Solid Edge part; units mm, degrees
sketch "Sketch1" plane through (0, 0, 0) normal (0, 0, 1) x (1, 0, 0)
  circle A0 centre (0, 0) radius 32
  circle A1 centre (0, 0) radius 21.1
  circle A2 centre (27, 0) radius 1.7
  circle A3 centre (0, 27) radius 1.7
  circle A4 centre (-27, 0) radius 1.7
  circle A5 centre (0, -27) radius 1.7
extrude "Protrusion1" add sketch "Sketch1" along normal blind 7.15
sketch "Sketch2" plane through (0, 0, 7.15) normal (0, 0, 1) x (1, 0, 0)
  circle A0 centre (0, 0) radius 32
  circle A1 centre (0, 0) radius 17.5
  circle A2 centre (27, 0) radius 1.7
  circle A3 centre (0, 27) radius 1.7
  circle A4 centre (-27, 0) radius 1.7
  circle A5 centre (0, -27) radius 1.7
extrude "ExtrudedProtrusion_2" add sketch "Sketch2" along normal blind 14.7
sketch "Sketch3" plane through (0, 0, 21.85) normal (0, 0, 1) x (1, 0, 0)
  circle A0 centre (0, 0) radius 32
  circle A1 centre (0, 0) radius 21.1
  circle A2 centre (27, 0) radius 1.7
  circle A3 centre (0, 27) radius 1.7
  circle A4 centre (-27, 0) radius 1.7
  circle A5 centre (0, -27) radius 1.7
extrude "ExtrudedProtrusion_3" add sketch "Sketch3" along normal blind 7.15
sketch "Sketch4" plane through (0, 0, 18.5) normal (0, 0, 1) x (1, 0, 0)
  circle A0 centre (0, 0) radius 42
  circle A1 centre (0, 0) radius 17.5
  circle A2 centre (27, 0) radius 1.7
  circle A3 centre (0, 27) radius 1.7
  circle A4 centre (-27, 0) radius 1.7
  circle A5 centre (0, -27) radius 1.7
  circle A6 centre (37, 0) radius 1.7
  circle A7 centre (0, 37) radius 1.7
  circle A8 centre (-37, 0) radius 1.7
  circle A9 centre (0, -37) radius 1.7
extrude "ExtrudedProtrusion_4" add sketch "Sketch4" along normal blind 5
For this review, take the finished solid that the model builds, in its own axes (mm). A direction names the side the tool comes from. Round coordinates to 2 decimals unless told otherwise and drop trailing zeros. Order: outer loops, then holes, each group sorted by start corner. A loop starts at its lowest first (then second) coordinate and runs counter-clockwise, first axis right, second up. Notation, with made-up numbers: M 58,-13.5 L 101,-13.5 A20 ccw 101,8.5 Z; hole C 44,83.5 d5. An arc over 180 degrees is marked long. Write each question's results on one line, items separated by ' | '. Start each with the question number.
1. Add section D-D (y = 0). State how many separate pieces and enclosed holes the cut face has, then the cut area to 3 significant figures.
2. Draft analysis for pull direction Y (two halves, no side actions). For faces 1 (the face through (20.126, -6.338, 3.525)), 2 (the face through (-6.94, 31.24, 9.12)), 3 (the face through (-8, 16, 7.15)), 4 (the face through (9, -31, 23.5)), state which applies: pulls with the +Y half, pulls with the -Y half, needs draft (parallel to the pull), parting line crosses it, or undercut.
3. Tool access review of faces 5 (the face through (9, -31, 18.5)), 6 (the face through (40.06, -12.62, 20.96)), 7 (the face through (20.126, -6.338, 26.212)): name each direction out of +Z, -Z, +X, -X, +Y, -Y from which nothing blocks a thin tool from reaching the whole face with its end or side.
4. Add section C-C (y = -27). State the section outline as (x, z) points, then the cut area to 3 significant figures.
5. Add section B-B (z = 12). State the section outline as (x, y) points, then the cut area to 3 significant figures.
6. Add section A-A (x = 8). State the section outline as (y, z) points, then the cut area to 3 significant figures.
7. To check wall thickness, follow L1, parallel to Y at x = 0, z = 20.95; L2, parallel to Y at x = 0, z = 1.75; L3, parallel to Y at x = 0, z = 17. State the ranges of each line that lie inside material, in increasing order. Write a range as [from, to].
8. Clearance check with flat-ended pins moving along their axes: pin 1 Ø5.5 at (x, y) = (-37, 0) entering from +Z; pin 2 Ø10 at (x, z) = (32.5, 5) entering from -Y; pin 3 Ø4 at (y, z) = (-26.5, 10) entering from -X. State where each tip first meets the part, or that it passes through.
Output values:
1) separate pieces: 6 | enclosed holes: 0 | area: 619 mm^2
2) face 1: undercut | face 2: parting line crosses it | face 3: undercut | face 4: needs draft
3) face 5: -Z | face 6: +Z, -Z | face 7: +Z
4) outline: M -32.17,18.5 L -17.18,18.5 L -17.18,0 L -1.7,0 L -1.7,29 L -17.18,29 L -17.18,23.5 L -32.17,23.5 Z; M 1.7,0 L 17.18,0 L 17.18,18.5 L 32.17,18.5 L 32.17,23.5 L 17.18,23.5 L 17.18,29 L 1.7,29 Z | area: 1,050 mm^2
5) outline: C 0,0 d64; hole C -27,0 d3.4; hole C 0,0 d35; hole C 0,-27 d3.4; hole C 0,27 d3.4; hole C 27,0 d3.4 | area: 2,220 mm^2
6) outline: M -41.23,18.5 L -30.98,18.5 L -30.98,0 L -19.52,0 L -19.52,7.15 L -15.56,7.15 L -15.56,23.5 L -19.52,23.5 L -19.52,29 L -30.98,29 L -30.98,23.5 L -41.23,23.5 Z; M 15.56,7.15 L 19.52,7.15 L 19.52,0 L 30.98,0 L 30.98,18.5 L 41.23,18.5 L 41.23,23.5 L 30.98,23.5 L 30.98,29 L 19.52,29 L 19.52,23.5 L 15.56,23.5 Z | area: 897 mm^2
7) L1: [-42, -38.7], [-35.3, -28.7], [-25.3, -17.5], [17.5, 25.3], [28.7, 35.3], [38.7, 42] | L2: [-32, -28.7], [-25.3, -21.1], [21.1, 25.3], [28.7, 32] | L3: [-32, -28.7], [-25.3, -17.5], [17.5, 25.3], [28.7, 32]
8) pin 1: z = 23.5 | pin 2: y = -16.36 | pin 3: x = -20.59
